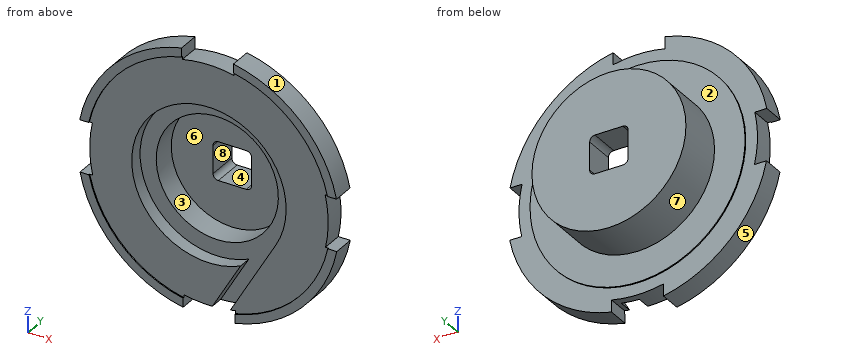
from build123d import *

# Parameters (mm, degrees)
SKETCH1_W           = 10
SKETCH1_H           = 10
BOSS_EXTRUDE2_DEPTH = 6
CUT_EXTRUDE1_DEPTH  = 3.81
SKETCH3_R           = 31.75
CUT_EXTRUDE2_DEPTH  = 0.3
SKETCH4_R           = 20.01
SKETCH4_W           = 10
SKETCH4_H           = 10
BOSS_EXTRUDE3_DEPTH = 12.065
SKETCH5_R           = 15.875
CUT_EXTRUDE3_DEPTH  = 6.35
FILLET1_R           = 1.3716
SKETCH6_R           = 54.970137174
SKETCH6_R_2         = 27.94
CUT_EXTRUDE4_DEPTH  = 0.3


with BuildPart() as part:
    # Sketch1 → Boss-Extrude2 (new body)
    with BuildSketch(Plane(origin=(0, 0, 0), x_dir=(1, 0, 0), z_dir=(0, 1, 0))):
        with BuildLine():
            Line((30.289899368, 6.5405), (33.401663967, 6.5405))
            ThreePointArc((33.401663967, 6.5405), (24.204111991, 23.929276184), (6.9215, 33.32479758))
            Line((6.9215, 33.32479758), (6.9215, 30.205115159))
            ThreePointArc((6.9215, 30.205115159), (0.195159782, 30.987385444), (-6.5405, 30.289899368))
            Line((-6.5405, 30.289899368), (-6.5405, 33.401663967))
            ThreePointArc((-6.5405, 33.401663967), (-23.929276184, 24.204111991), (-33.32479758, 6.9215))
            Line((-33.32479758, 6.9215), (-30.205115159, 6.9215))
            ThreePointArc((-30.205115159, 6.9215), (-30.987385444, 0.195159782), (-30.289899368, -6.5405))
            Line((-30.289899368, -6.5405), (-33.401663967, -6.5405))
            ThreePointArc((-33.401663967, -6.5405), (-24.204111991, -23.929276184), (-6.9215, -33.32479758))
            Line((-6.9215, -33.32479758), (-6.9215, -30.205115159))
            ThreePointArc((-6.9215, -30.205115159), (-0.195159782, -30.987385444), (6.5405, -30.289899368))
            Line((6.5405, -30.289899368), (6.5405, -33.401663967))
            ThreePointArc((6.5405, -33.401663967), (23.929276184, -24.204111991), (33.32479758, -6.9215))
            Line((33.32479758, -6.9215), (30.205115159, -6.9215))
            ThreePointArc((30.205115159, -6.9215), (30.987385444, -0.195159782), (30.289899368, 6.5405))
        make_face()
        Rectangle(SKETCH1_W, SKETCH1_H, mode=Mode.SUBTRACT)
    extrude(amount=BOSS_EXTRUDE2_DEPTH)

    # Sketch2 → Cut-Extrude1 (cut)
    with BuildSketch(Plane.XZ):
        with BuildLine():
            Line((17.377665752, -10.033), (-0.286554615, -40.628327152))
            ThreePointArc((-0.286554615, -40.628327152), (-2.416432138, -40.557415308), (-4.539661745, -40.374924792))
            Line((-4.539661745, -40.374924792), (8.196212586, -18.315743371))
            ThreePointArc((8.196212586, -18.315743371), (-13.440862054, 14.899247741), (17.377665752, -10.033))
        make_face()
    extrude(amount=-CUT_EXTRUDE1_DEPTH, mode=Mode.SUBTRACT)

    # Sketch3 → Cut-Extrude2 (cut)
    with BuildSketch(Plane.XZ):
        Circle(SKETCH3_R)
    extrude(amount=-CUT_EXTRUDE2_DEPTH, mode=Mode.SUBTRACT)

    # Sketch4 → Boss-Extrude3 (add)
    with BuildSketch(Plane(origin=(0, 6, 0), x_dir=(1, 0, 0), z_dir=(0, 1, 0))):
        with Locations(Location((0, 0, 0), (0, 0, 90))):
            Circle(SKETCH4_R)
        Rectangle(SKETCH4_W, SKETCH4_H, mode=Mode.SUBTRACT)
    extrude(amount=BOSS_EXTRUDE3_DEPTH)

    # Sketch5 → Cut-Extrude3 (cut)
    with BuildSketch(Plane.XZ.offset(-3.81)):
        with Locations(Location((0, 0, 0), (0, 0, 270))):
            Circle(SKETCH5_R)
    extrude(amount=-CUT_EXTRUDE3_DEPTH, mode=Mode.SUBTRACT)

    # Fillet1
    fillet1_edges = [part.edges().sort_by_distance(p)[0] for p in [
        (5, 14.1125, -5),
        (-5, 14.1125, -5),
        (-5, 14.1125, 5),
        (5, 14.1125, 5),
    ]]
    fillet(fillet1_edges, radius=FILLET1_R)

    # Sketch6 → Cut-Extrude4 (cut)
    with BuildSketch(Plane(origin=(0, 6, 0), x_dir=(1, 0, 0), z_dir=(0, 1, 0))):
        Circle(SKETCH6_R)
        with Locations(Location((0, 0, 0), (0, 0, 270))):
            Circle(SKETCH6_R_2, mode=Mode.SUBTRACT)
    extrude(amount=-CUT_EXTRUDE4_DEPTH, mode=Mode.SUBTRACT)


solid = part.part
Verification items for the finished model (mm, model axes). Face numbers are marked on the shaded views. A direction names the side the tool comes from. Give positions to 0.01 mm unless a question says otherwise; leave off trailing zeros. Write each loop counter-clockwise with the first axis right and the second up, starting at its lowest first coordinate (ties: lowest second). Pieces come first, ordered by that corner, then holes. Notation, with made-up numbers: M 43.25,27 L 57.25,27 A18 cw 57.25,62 Z; hole C 2,80.25 d7. An arc over 180 degrees is marked long. Use CSV: the item, a comma, the result in double quotes.
1) Release check for a two-part mould opening along Z. For the marked faces 1, 2, 3 and 4 record: released by +Z, released by -Z, zero draft, split by the parting line, or undercut.
Final values:
face 1,"released by +Z"
face 2,"zero draft"
face 3,"undercut"
face 4,"undercut"
2) Cross-section at B-B (z = 0). Enter the section's corners in (x, y) (3 decimals), plus the area to 3 significant figures.
Final values:
outline,"M -30.988,0.3 L -20.066,0.3 L -20.066,3.81 L -15.875,3.81 L -15.875,10.16 L -5,10.16 L -5,18.065 L -20.01,18.065 L -20.01,6 L -27.94,6 L -27.94,5.7 L -30.988,5.7 Z; M 5,10.16 L 15.875,10.16 L 15.875,3.81 L 20.066,3.81 L 20.066,0.3 L 30.988,0.3 L 30.988,5.7 L 27.94,5.7 L 27.94,6 L 20.01,6 L 20.01,18.065 L 5,18.065 Z"
area,"413 mm²"
3) Cross-section at C-C (y = 13). Enter the section's corners in (x, z), plus the area to 3 significant figures.
Final values:
outline,"C 0,0 d40.02; hole M -5,-3.63 A1.37 ccw -3.63,-5 L 3.63,-5 A1.37 ccw 5,-3.63 L 5,3.63 A1.37 ccw 3.63,5 L -3.63,5 A1.37 ccw -5,3.63 Z"
area,"1,160 mm²"
4) Access from +Z, -Z, +X, -X, +Y, -Y to the whole of each face (thin tool, end or side, straight path). Record for the marked faces 5, 6, 7 and 8.
Final values:
face 5,"-Z, -X, +Y, -Y"
face 6,"-Y"
face 7,"+Y"
face 8,"+Y, -Y"
5) Cross-section at D-D (z = 11.5). Enter the section's corners in (x, y) (3 decimals), plus the area to 3 significant figures.
Final values:
outline,"M -32.034,0 L -29.594,0 L -29.594,0.3 L -16.444,0.3 L -16.444,3.81 L -10.944,3.81 L -10.944,10.16 L 10.944,10.16 L 10.944,3.81 L 16.444,3.81 L 16.444,0.3 L 29.594,0.3 L 29.594,0 L 32.034,0 L 32.034,5.7 L 25.464,5.7 L 25.464,6 L 16.375,6 L 16.375,18.065 L -16.375,18.065 L -16.375,6 L -25.464,6 L -25.464,5.7 L -32.034,5.7 Z"
area,"503 mm²"
6) Go/stop test with flat-tipped pins: pin 1 Ø1.6 at (y, z) = (3, 32) entering from +X; pin 2 Ø1.6 at (x, y) = (32, 4) entering from +Z; pin 3 Ø8 at (y, z) = (14.5, 1.5) entering from +X. Record where each tip stops, or that it passes through.
Final values:
pin 1,"x = 13.6"
pin 2,"z = 13.6"
pin 3,"x = 20.01"
7) Material ranges on line 1 along X through (y, z) = (2.05, 0); line 2 along Z through (x, y) = (0.5, 11.5), recorded low to high.
Final values:
line 1,"-30.99 to -20.07, 20.07 to 30.99"
line 2,"-20 to -5, 5 to 20"
8) Cross-section at A-A (x = 0). Enter the section's corners in (y, z) (3 decimals).
Final values:
outline,"M 0.3,-30.988 L 5.7,-30.988 L 5.7,-27.94 L 6,-27.94 L 6,-20.01 L 18.065,-20.01 L 18.065,-5 L 10.16,-5 L 10.16,-15.875 L 3.81,-15.875 L 3.81,-20.066 L 0.3,-20.066 Z; M 0.3,20.066 L 3.81,20.066 L 3.81,15.875 L 10.16,15.875 L 10.16,5 L 18.065,5 L 18.065,20.01 L 6,20.01 L 6,27.94 L 5.7,27.94 L 5.7,30.988 L 0.3,30.988 Z"
